The listing builds one solid part. Answer for the finished solid, in the listing's coordinates (mm). A direction names the side the tool comes from. Give positions to 0.01 mm unless a question says otherwise; leave off trailing zeros. Write each loop counter-clockwise with the first axis right and the second up, starting at its lowest first coordinate (ties: lowest second). Pieces come first, ordered by that corner, then holes. Notation, with made-up numbers: (6.25, 24.5) - (44.25, 24.5) arc R18 ccw to (44.25, 31.5) - close; hole circle Ø6 at (23, 76.5). An arc over 180 degrees is marked (long way). One line per question, with ' | ' between items. Start each with the question number.
1. A cutting plane is placed at C-C (z = -17). Determine the outline of the cut face in (x, y).
2. A cutting plane is placed at A-A (x = 0). Determine the outline of the cut face in (y, z).
3. A cutting plane is placed at D-D (x = -7). Determine the outline of the cut face in (y, z), then the cut area to 3 significant figures.
4. Find the intervals of material crossed by L1, parallel to Y at x = -11, z = 0; L2, parallel to X at y = 9, z = 0; L3, parallel to Z at x = 3.5, y = 1.5, in increasing order. Write a range as from..to.
5. A cutting plane is placed at B-B (z = 0). Determine the outline of the cut face in (x, y), then the cut area to 3 significant figures.
6. Given P1, Ø4, axis at x = 17.34, z = 16.36, coming from the -Y side; P2, Ø12, axis at x = 5.5, y = 17.5, coming from the +Z side; P3, Ø4.5, axis at y = 17.55, z = 0, coming from the +X side; P4, Ø2, axis at y = 19, z = -10, coming from the -X side, each flat-ended and moving along its own axis, determine where each tip first touches the part or whether it passes through.
7. For faces 1 (the face through (14, 11, 6)), 2 (the face through (-11.52, 13.79, 0.83)), 3 (the face through (-19.62, 5.58, -16.06)), determine the directions among +Z, -Z, +X, -X, +Y, -Y from which every point of the face is accessible in a straight line to the end or side of a thin tool.
8. The mould has two halves that part along X. Classify faces 4 (the face through (7, 0, 6)), 5 (the face through (22.14, 5.58, -9.03)), 6 (the face through (1.32, 5.42, -29.97)): +X half, -X half, draft (parallel to the pull), parting line (faces both ways), or undercut.
```python
from build123d import *

# Parameters (mm, degrees)
SKETCH2_R               = 15
BOSS_EXTRUDE1_DEPTH     = 26
SKETCH1_R               = 30
BOSS_EXTRUDE2_DEPTH     = 11
SKETCH3_R               = 9
CUT_EXTRUDE1_DEPTH      = 50.759421218
SKETCH4_R               = 2.3
CUT_EXTRUDE2_DEPTH      = 46
CIRPATTERN1_COUNT       = 6
CUT_EXTRUDE3_REACH      = 51.759
CUT_EXTRUDE3_END_RADIUS = 15
SKETCH7_R               = 3.85


with BuildPart() as part:
    # Sketch2 → Boss-Extrude1 (new body)
    with BuildSketch(Plane(origin=(0, 0, 0), x_dir=(1, 0, 0), z_dir=(0, 1, 0))):
        with Locations(Location((0, 0, 0), (0, 0, 270))):
            Circle(SKETCH2_R)
    extrude(amount=BOSS_EXTRUDE1_DEPTH)

    # Sketch1 → Boss-Extrude2 (add)
    with BuildSketch(Plane(origin=(0, 0, 0), x_dir=(1, 0, 0), z_dir=(0, 1, 0))):
        with Locations(Location((0, 0, 0), (0, 0, 270))):
            Circle(SKETCH1_R)
    extrude(amount=BOSS_EXTRUDE2_DEPTH)

    # Sketch3 → Cut-Extrude1 (cut, through all)
    with BuildSketch(Plane(origin=(0, 26, 0), x_dir=(1, 0, 0), z_dir=(0, 1, 0))):
        with Locations(Location((0, 0, 0), (0, 0, 270))):
            Circle(SKETCH3_R)
    extrude(amount=-CUT_EXTRUDE1_DEPTH, mode=Mode.SUBTRACT)

    # Sketch4 → Cut-Extrude2 (cut, through all)
    with BuildSketch(Plane(origin=(0, 11, 0), x_dir=(1, 0, 0), z_dir=(0, 1, 0))):
        with Locations(Location((5.495034326, 23.192449843, 0), (0, 0, 270))):
            Circle(SKETCH4_R)
    cut_extrude2 = extrude(amount=-CUT_EXTRUDE2_DEPTH, mode=Mode.SUBTRACT)

    # CirPattern1: Cut-Extrude2 ×6 about axis
    cirpattern1_axis = Axis((0, 0, 0), (0, 1, 0))
    for i in range(1, CIRPATTERN1_COUNT):
        add(cut_extrude2.rotate(cirpattern1_axis, i * 360 / CIRPATTERN1_COUNT), mode=Mode.SUBTRACT)

    # Cut-Extrude3: up to this cylinder (the profile starts inside it)
    cut_extrude3_end = Plane(origin=(0, 17.55, 0), z_dir=(0, -1, 0)) * Cylinder(CUT_EXTRUDE3_END_RADIUS, 134.518, mode=Mode.PRIVATE)
    # Sketch7 → Cut-Extrude3 (cut, up to the surface)
    with BuildSketch(Plane(origin=(0, 0, 0), x_dir=(0, 0, -1), z_dir=(1, 0, 0)), mode=Mode.PRIVATE) as cut_extrude3_sk1:
        with Locations((0, 17.55)):
            Circle(SKETCH7_R)
    cut_extrude3_tool1 = extrude(cut_extrude3_sk1.sketch, amount=-CUT_EXTRUDE3_REACH, mode=Mode.PRIVATE) & cut_extrude3_end
    add(cut_extrude3_tool1.solids().sort_by_distance((0, 17.55, 0))[0], mode=Mode.SUBTRACT)


solid = part.part
```
Determined:
1) outline: (-24.72, 0) - (-19.55, 0) - (-19.55, 11) - (-24.72, 11) - close; (-15.13, 0) - (24.72, 0) - (24.72, 11) - (-15.13, 11) - close
2) outline: (0, -30) - (11, -30) - (11, -15) - (26, -15) - (26, -9) - (0, -9) - close; (0, 9) - (26, 9) - (26, 15) - (11, 15) - (11, 30) - (0, 30) - close
3) outline: (0, -29.17) - (11, -29.17) - (11, -13.27) - (26, -13.27) - (26, -5.66) - (0, -5.66) - close; (0, 5.66) - (26, 5.66) - (26, 13.27) - (11, 13.27) - (11, 21.45) - (0, 21.45) - close; (0, 24.93) - (11, 24.93) - (11, 29.17) - (0, 29.17) - close | area: 707 mm2
4) L1: 0..13.7, 21.4..26 | L2: -30..-9, 9..30 | L3: -29.8..-24.34, -22.05..-8.29, 8.29..29.8
5) outline: (-30, 0) - (-9, 0) - (-9, 13.7) - (-15, 13.7) - (-15, 11) - (-30, 11) - close; (-15, 21.4) - (-9, 21.4) - (-9, 26) - (-15, 26) - close; (9, 0) - (30, 0) - (30, 11) - (15, 11) - (15, 26) - (9, 26) - close | area: 596 mm2
6) P1: through | P2: z = 15 | P3: x = 15 | P4: x = -12
7) face 1: +Y | face 2: -X | face 3: +Y, -Y
8) face 4: draft | face 5: undercut | face 6: parting line
